Build history of the part. All positions in model axes, mm. Face numbers are marked on the shaded views. A direction names the side the tool comes from. Give positions to 0.01 mm unless a question says otherwise; leave off trailing zeros. Write each loop counter-clockwise with the first axis right and the second up, starting at its lowest first coordinate (ties: lowest second). Pieces come first, ordered by that corner, then holes. Notation, with made-up numbers: (89.25, 48.5) -> (144.25, 48.5) arc R16 cw to (144.25, 62.5) -> close; hole circle Ø7 at (0.5, 66.5). An arc over 180 degrees is marked (long way). Put each result on its own line as item: value.
from build123d import *

# Parameters (mm, degrees)
SKETCH_1_R      = 30
SKETCH_1_W      = 35
SKETCH_1_H      = 35
EXTRUDE_1_DEPTH = 100


with BuildPart() as part:
    # 草图1 → 凸台-拉伸1 (new body)
    with BuildSketch(Plane.XY):
        with Locations((17.5, 17.5)):
            Circle(SKETCH_1_R)
        with Locations((17.5, 17.5)):
            Rectangle(SKETCH_1_W, SKETCH_1_H, mode=Mode.SUBTRACT)
    extrude(amount=EXTRUDE_1_DEPTH)


solid = part.part
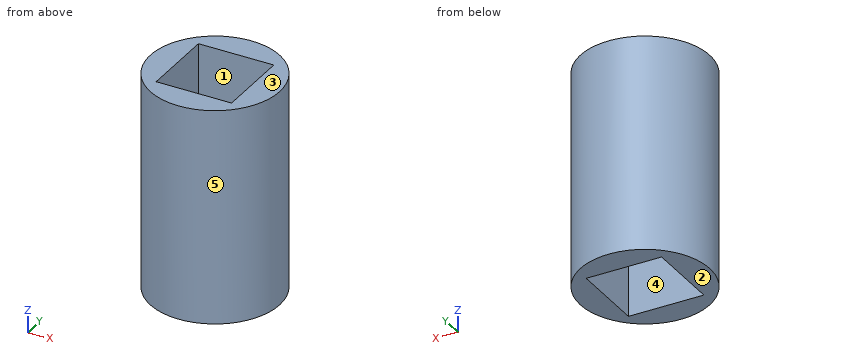
1) Slice it at C-C (z = 67). Write the cut outline in (x, y), plus the area to 3 significant figures.
Filled sheet:
outline: circle Ø60 at (17.5, 17.5); hole (0, 0) -> (35, 0) -> (35, 35) -> (0, 35) -> close
area: 1,600 mm2
2) Pin check, flat tips, straight feed: pin 1 (6 mm diameter, centred on y = 3, z = 56, fed in from +X); pin 2 (1.5 mm diameter, centred on y = 10, z = 55.5, fed in from -X); pin 3 (1.5 mm diameter, centred on x = 21.5, z = 62, fed in from +Y). Stop position of each tip, or through.
Filled sheet:
pin 1: x = 45.21
pin 2: x = -11.73
pin 3: y = 47.32
3) Slice it at D-D (y = 37.5). Write the cut outline in (x, z).
Filled sheet:
outline: (-4.86, 0) -> (39.86, 0) -> (39.86, 100) -> (-4.86, 100) -> close
4) Pull direction Y, two halves, no side cores. Call the marked faces 3, 4 and 5: released by +Y, released by -Y, zero draft, split by the parting line, or undercut.
Filled sheet:
face 3: zero draft
face 4: undercut
face 5: split by the parting line
5) Wall check: L1, parallel to Y at x = 18, z = 18; L2, parallel to X at y = 21, z = 10. Give the ranges that are in metal, low to high.
Filled sheet:
L1: -12.5 to 0, 35 to 47.5
L2: -12.3 to 0, 35 to 47.3
6) Slice it at A-A (y = 17.5). Write the cut outline in (x, z).
Filled sheet:
outline: (-12.5, 0) -> (0, 0) -> (0, 100) -> (-12.5, 100) -> close; (35, 0) -> (47.5, 0) -> (47.5, 100) -> (35, 100) -> close
7) Tool access for the marked faces 1 and 2: list every direction of +Z, -Z, +X, -X, +Y, -Y with a clear straight run to the whole face (end or side of a thin tool).
Filled sheet:
face 1: +Z, -Z
face 2: -Z, +X, -X, +Y, -Y
